Read the model definition and answer for the solid it produces. Units are mm, in the model's axes. Give positions to 0.01 mm unless a question says otherwise; leave off trailing zeros. Order: outer loops, then holes, each group sorted by start corner. A loop starts at its lowest first (then second) coordinate and runs counter-clockwise, first axis right, second up. Notation, with made-up numbers: M 41,59.25 L 77,59.25 A20 cw 77,92.25 Z; hole C 36,38 d7. An arc over 180 degrees is marked long. One line per item, written item: value.
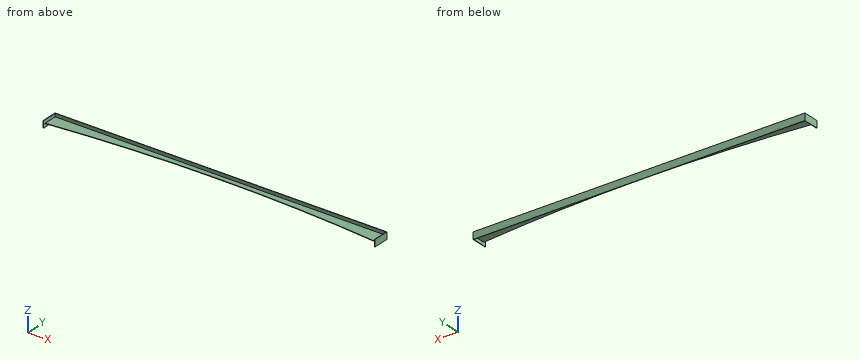
from build123d import *

# Parameters (mm, degrees)
BOSS_EXTRUDE1_DEPTH = 19.05
RIB1_START          = -1.27
RIB1_DEPTH          = 2.54


# Read off the part's stored shape, not the designer's step: Rib1
with BuildPart() as part:
    # Sketch1 → Boss-Extrude1 (new, symmetric)
    with BuildSketch(Plane.XY):
        Polygon((-921.54375, 88.9), (921.54375, 88.9), (921.54375, 0), (919.00375, 0), (919.00375, 86.36), (-919.00375, 86.36), (-919.00375, 0), (-921.54375, 0), align=None)
    extrude(amount=BOSS_EXTRUDE1_DEPTH, both=True)

    # Rib1 outline → Rib1 (add)
    with BuildSketch(Plane.XY.offset(RIB1_START)):
        with BuildLine():
            Line((-919.00375, 86.36), (-919.00375, 12.7))
            ThreePointArc((-919.00375, 12.7), (0, 60.96), (919.00375, 12.7))
            Line((919.00375, 12.7), (919.00375, 86.36))
            Line((919.00375, 86.36), (-919.00375, 86.36))
        make_face()
    extrude(amount=RIB1_DEPTH)


solid = part.part
1) Each of these flat-tipped pins is pushed along its axis until it touches: pin 1 Ø12 at (x, z) = (144.5, -12) entering from -Y; pin 2 Ø6 at (x, y) = (-545, 78) entering from +Z; pin 3 Ø1 at (x, y) = (192, 80) entering from -Z. Where does it stop, or does it pass through?
Reported:
pin 1: stops at y = 86.36
pin 2: stops at z = 1.27
pin 3: stops at z = -1.27
2) Find section C-C, the plane x = 444. Write down the section's boundary in (y, z), plus the area to 3 significant figures.
Reported:
outline: M 49.72,-1.27 L 86.36,-1.27 L 86.36,-19.05 L 88.9,-19.05 L 88.9,19.05 L 86.36,19.05 L 86.36,1.27 L 49.72,1.27 Z
area: 190 mm^2
3) Consider probe 1 along X at (y, z) = (38, -10); probe 2 along Y at (x, z) = (814.5, 17); probe 3 along Z at (x, y) = (765, 76.5). Determine where each line is inside the solid, lowest interval first.
Reported:
probe 1: x = -921.54 to -919, 919 to 921.54
probe 2: y = 86.36 to 88.9
probe 3: z = -1.27 to 1.27
4) Find section A-A, the plane y = 43.5. Write down the section's boundary in (x, z).
Reported:
outline: M -921.54,-19.05 L -919,-19.05 L -919,-1.27 L -553.26,-1.27 L -553.26,1.27 L -919,1.27 L -919,19.05 L -921.54,19.05 Z; M 553.26,-1.27 L 919,-1.27 L 919,-19.05 L 921.54,-19.05 L 921.54,19.05 L 919,19.05 L 919,1.27 L 553.26,1.27 Z
5) Find section B-B, the plane z = -10. Write down the section's boundary in (x, y).
Reported:
outline: M -921.54,0 L -919,0 L -919,86.36 L 919,86.36 L 919,0 L 921.54,0 L 921.54,88.9 L -921.54,88.9 Z
